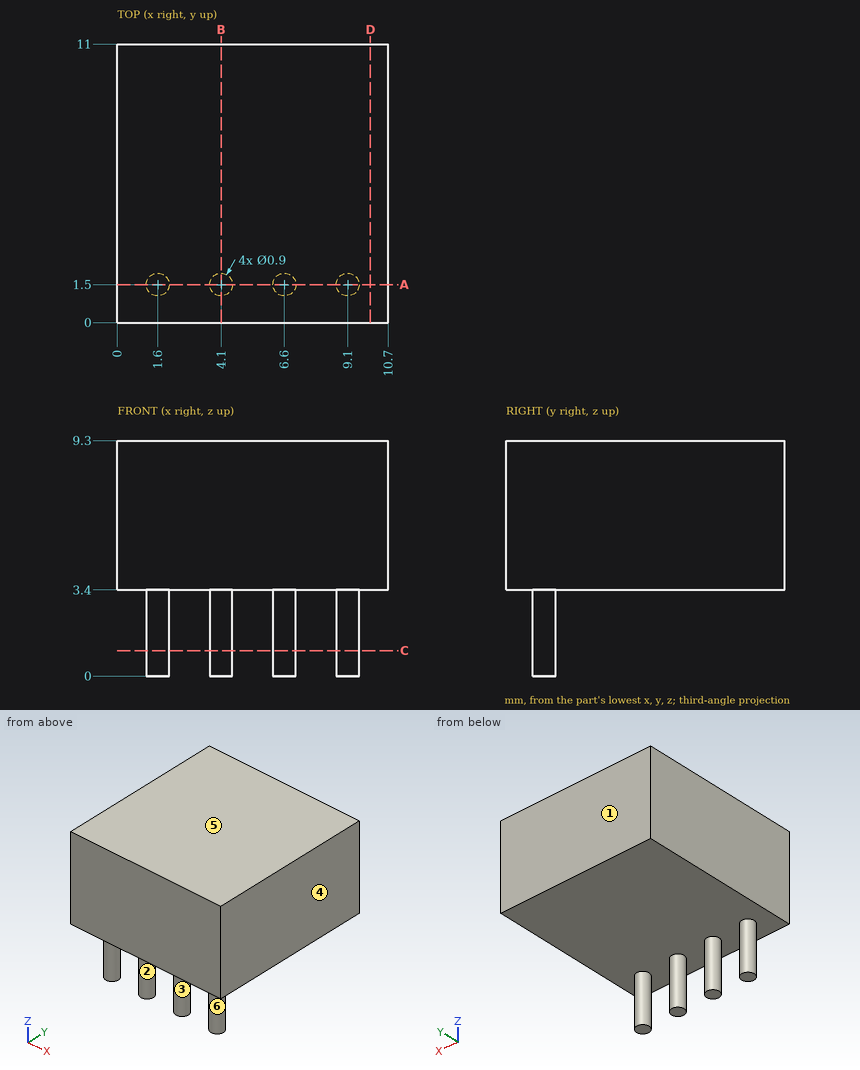
Verification items for this drawing (mm, ordinates from the low corner). A direction names the side the tool comes from. Round coordinates to 2 decimals unless told otherwise and drop trailing zeros. Loops run counter-clockwise (first coordinate to the right, second up) from the corner with the lowest first, then second, coordinate; pieces in that order, holes last. Notation, with made-up numbers: M -37,32 L 11,32 A6 cw 11,38 Z; hole C -37,-13.75 d11. An arc over 180 degrees is marked long. Answer as a JSON object with one key per item and string values.
1. Section check A-A (y = 1.5). Record the boundary of the cut face in (x, z), plus the area to 3 significant figures.
Reply:
{"outline": "M 0,3.4 L 1.15,3.4 L 1.15,0 L 2.05,0 L 2.05,3.4 L 3.65,3.4 L 3.65,0 L 4.55,0 L 4.55,3.4 L 6.15,3.4 L 6.15,0 L 7.05,0 L 7.05,3.4 L 8.65,3.4 L 8.65,0 L 9.55,0 L 9.55,3.4 L 10.7,3.4 L 10.7,9.3 L 0,9.3 Z", "area": "75.4 mm²"}
2. Section check D-D (x = 10). Record the boundary of the cut face in (y, z), plus the area to 3 significant figures.
Reply:
{"outline": "M 0,3.4 L 11,3.4 L 11,9.3 L 0,9.3 Z", "area": "64.9 mm²"}
3. Access from +Z, -Z, +X, -X, +Y, -Y to the whole of each face (thin tool, end or side, straight path). Record for the marked faces 1 and 2.
Reply:
{"face 1": "+Z, -Z, +X, -X, +Y", "face 2": "-Z"}
4. Mould release check, pull along X, two halves, no side actions. Record for the marked faces 3, 4, 5 and 6: pulls with the +X half, pulls with the -X half, needs draft (parallel to the pull), parting line crosses it, or undercut.
Reply:
{"face 3": "undercut", "face 4": "pulls with the +X half", "face 5": "needs draft", "face 6": "undercut"}
5. Section check C-C (z = 1). Record the boundary of the cut face in (x, y), plus the area to 3 significant figures.
Reply:
{"outline": "C 1.6,1.5 d0.9; C 4.1,1.5 d0.9; C 6.6,1.5 d0.9; C 9.1,1.5 d0.9", "area": "2.54 mm²"}
6. Gauge pin test, flat end, axial feed: P1, Ø2, axis at y = 7.5, z = 1, coming from the -X side. Record the tip position at first contact, or that the pin passes through.
Reply:
{"P1": "passes through"}
7. Section check B-B (x = 4.1). Record the boundary of the cut face in (y, z), plus the area to 3 significant figures.
Reply:
{"outline": "M 0,3.4 L 1.05,3.4 L 1.05,0 L 1.95,0 L 1.95,3.4 L 11,3.4 L 11,9.3 L 0,9.3 Z", "area": "68.0 mm²"}
8. Scan line: line 1 (Z direction, x = 6.75, y = 9). Record every from-to range of solid material in increasing order.
Reply:
{"line 1": "z = 3.4 to 9.3"}
